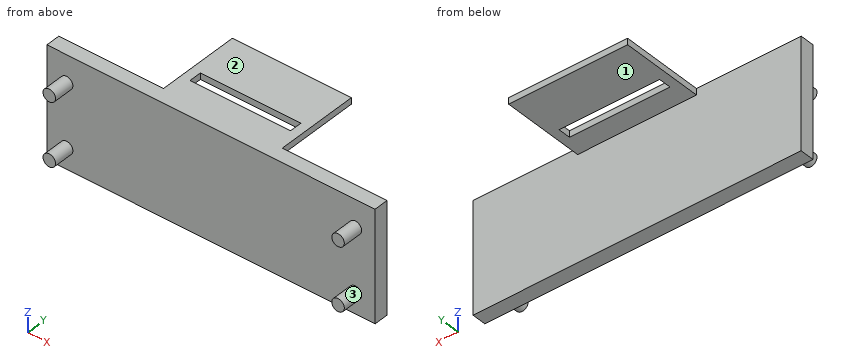
from build123d import *

# Parameters (mm, degrees)
SKETCH1_W           = 56.807908868
SKETCH1_H           = 54.266272082
BOSS_EXTRUDE2_DEPTH = 3
SKETCH2_R           = 4.25
BOSS_EXTRUDE3_DEPTH = 12
SKETCH3_W           = 48
SKETCH3_H           = 6
CUT_EXTRUDE1_DEPTH  = 10
SKETCH4_W           = 56.807908868
SKETCH4_H           = 6.889223191
BOSS_EXTRUDE4_DEPTH = 50
SKETCH5_W           = 53
SKETCH5_H           = 6.889223191
BOSS_EXTRUDE5_DEPTH = 50
SKETCH8_W           = 53
SKETCH8_H           = 6.889223191
BOSS_EXTRUDE6_DEPTH = 50
SKETCH9_W           = 68.867558101
SKETCH9_H           = 60.331860759
CUT_EXTRUDE2_DEPTH  = 26
SKETCH10_W          = 129.878394785
SKETCH10_H          = 53.736094631
CUT_EXTRUDE3_DEPTH  = 22
BOSS_EXTRUDE7_START = -6.889223
SKETCH11_R          = 3
BOSS_EXTRUDE7_DEPTH = 10


with BuildPart() as part:
    # Sketch1 → Boss-Extrude2 (new body)
    with BuildSketch(Plane.XY):
        with Locations((-6.025526457, -12.157362225)):
            Rectangle(SKETCH1_W, SKETCH1_H)
    extrude(amount=-BOSS_EXTRUDE2_DEPTH)

    # Sketch2 → Boss-Extrude3 (add)
    with BuildSketch(Plane.XY):
        with Locations((-26.141196849, 5.26708344)):
            Circle(SKETCH2_R)
        with Locations((-6.541196849, 5.26708344)):
            Circle(SKETCH2_R)
        with Locations((13.058803151, 5.26708344)):
            Circle(SKETCH2_R)
        with Locations((-26.141196849, -29.58291656)):
            Circle(SKETCH2_R)
        with Locations((-6.541196849, -29.58291656)):
            Circle(SKETCH2_R)
        with Locations((13.058803151, -29.58291656)):
            Circle(SKETCH2_R)
    extrude(amount=BOSS_EXTRUDE3_DEPTH)

    # Sketch3 → Cut-Extrude1 (cut)
    with BuildSketch(Plane.XY):
        with Locations((-6.025526457, -11.783671744)):
            Rectangle(SKETCH3_W, SKETCH3_H)
    extrude(amount=-CUT_EXTRUDE1_DEPTH, mode=Mode.SUBTRACT)

    # Sketch4 → Boss-Extrude4 (add)
    with BuildSketch(Plane(origin=(0, 0, -3), x_dir=(-1, 0, 0), z_dir=(0, 0, -1))):
        with Locations((6.025526457, -28.22828334)):
            Rectangle(SKETCH4_W, SKETCH4_H)
    extrude(amount=BOSS_EXTRUDE4_DEPTH)

    # Sketch5 → Boss-Extrude5 (add)
    with BuildSketch(Plane(origin=(22.378427977, 0, 0), x_dir=(0, 0, -1), z_dir=(1, 0, 0))):
        with Locations((26.5, -28.22828334)):
            Rectangle(SKETCH5_W, SKETCH5_H)
    extrude(amount=BOSS_EXTRUDE5_DEPTH)

    # Sketch8 → Boss-Extrude6 (add)
    with BuildSketch(Plane.ZY.offset(34.429480891)):
        with Locations((-26.5, -28.22828334)):
            Rectangle(SKETCH8_W, SKETCH8_H)
    extrude(amount=BOSS_EXTRUDE6_DEPTH)

    # Sketch9 → Cut-Extrude2 (cut)
    with BuildSketch(Plane.XY):
        with Locations((-7.965457672, -13.030331271)):
            Rectangle(SKETCH9_W, SKETCH9_H)
    extrude(amount=CUT_EXTRUDE2_DEPTH, mode=Mode.SUBTRACT)

    # Sketch10 → Cut-Extrude3 (cut)
    with BuildSketch(Plane.XZ.offset(31.672894935)):
        with Locations((-14.803715202, -13.978089422)):
            Rectangle(SKETCH10_W, SKETCH10_H)
    extrude(amount=CUT_EXTRUDE3_DEPTH, mode=Mode.SUBTRACT)

    # Sketch11 → Boss-Extrude7 (add)
    with BuildSketch(Plane(origin=(0, -24.783671744, 0), x_dir=(1, 0, 0), z_dir=(0, 1, 0)).offset(BOSS_EXTRUDE7_START)):
        with Locations(Location((-75.025526457, 43, 0), (0, 0, 270))):
            Circle(SKETCH11_R)
        with Locations(Location((-75.025526457, 13, 0), (0, 0, 270))):
            Circle(SKETCH11_R)
        with Locations(Location((62.974473543, 13, 0), (0, 0, 270))):
            Circle(SKETCH11_R)
        with Locations(Location((62.974473543, 43, 0), (0, 0, 270))):
            Circle(SKETCH11_R)
    extrude(amount=-BOSS_EXTRUDE7_DEPTH)


solid = part.part
Model file for the job. Use its own axes, mm. Face numbers are marked on the shaded views. Round coordinates to 2 decimals unless told otherwise and drop trailing zeros. Loops run counter-clockwise (first coordinate to the right, second up) from the corner with the lowest first, then second, coordinate; pieces in that order, holes last.
1. Band-saw the part on A-A, the plane x = 13. List the corners of the cut face in (y, z), and give its area (3 significant figures).
Check values:
outline: (-31.67, -53) - (-24.78, -53) - (-24.78, -3) - (-14.78, -3) - (-14.78, 0) - (-31.67, 0) - close; (-8.78, -3) - (14.98, -3) - (14.98, 0) - (-8.78, 0) - close
area: 466 mm2
2. Band-saw the part on C-C, the plane y = 1. List the corners of the cut face in (x, z).
Check values:
outline: (-34.43, -3) - (22.38, -3) - (22.38, 0) - (-34.43, 0) - close
3. Mould opens along Z. For the marked faces 1, 2 and 3 say: +Z half, -Z half, draft (parallel to the pull), parting line (faces both ways), or undercut.
Check values:
face 1: -Z half
face 2: +Z half
face 3: undercut
4. Band-saw the part on D-D, the plane x = -69.5. List the corners of the cut face in (y, z), and give its area (3 significant figures).
Check values:
outline: (-31.67, -53) - (-24.78, -53) - (-24.78, 0) - (-31.67, 0) - close
area: 365 mm2
5. Band-saw the part on B-B, the plane z = -43. List the corners of the cut face in (x, y).
Check values:
outline: (-84.43, -31.67) - (-78.03, -31.67) - (-78.03, -41.67) - (-72.03, -41.67) - (-72.03, -31.67) - (59.97, -31.67) - (59.97, -41.67) - (65.97, -41.67) - (65.97, -31.67) - (72.38, -31.67) - (72.38, -24.78) - (-84.43, -24.78) - close
6. Wall check: probe 1 along Z at (x, y) = (-21, 6); probe 2 along Y at (x, z) = (-65, -4). Give the ranges that are in metal, low to high.
Check values:
probe 1: z = -3 to 0
probe 2: y = -31.67 to -24.78
7. Drop flat-ended pins along their axis: P1, Ø3, axis at x = -45, z = -18.5, coming from the +Y side; P2, Ø0.9, axis at y = -11.5, z = -1.5, coming from the +X side; P3, Ø6, axis at x = 12, y = -21.5, coming from the +Z side; P4, Ø20, axis at x = -9, y = -14, coming from the -Z side. Give the stop position or say it passes through.
Check values:
P1: stops at y = -24.78
P2: stops at x = 22.38
P3: stops at z = 0
P4: stops at z = -3
